Part model, mm, in its own coordinate system. Face numbers are marked on the shaded views. A direction names the side the tool comes from. Round coordinates to 2 decimals unless told otherwise and drop trailing zeros. Write each loop counter-clockwise with the first axis right and the second up, starting at its lowest first coordinate (ties: lowest second). Pieces come first, ordered by that corner, then holes. Notation, with made-up numbers: (-29, 78.5) -> (7, 78.5) arc R18 cw to (7, 104.5) -> close; hole circle Ø9 at (48, 11.25). An arc over 180 degrees is marked (long way). Return JSON: item names as keys, results as strings. Group by question number.
Autodesk Inventor part; units mm, degrees
ref_plane "YZ Plane" through (0, 0, 0) normal (1, 0, 0) x (0, 1, 0)
ref_plane "XZ Plane" through (0, 0, 0) normal (0, 1, 0) x (-1, 0, 0)
ref_plane "XY Plane" through (0, 0, 0) normal (0, 0, 1) x (1, 0, 0)
sketch "Эскиз1" plane through (0, 0, 0) normal (0, 1, 0) x (-1, 0, 0)
  line L0 (-40, 10) -> (40, 10)
  line L1 (40, 10) -> (40, -10)
  line L2 (40, -10) -> (-40, -10)
  line L3 (-40, -10) -> (-40, 10)
  line L4 (-40, 10) -> (40, -10) construction
  line L5 (40, 10) -> (-40, -10) construction
  point P0 (0, 0)
  dimension "d0" = 80
  dimension "d1" = 20
extrude "Выдавливание1" add sketch "Эскиз1" along normal blind 1.6
sketch "Эскиз2" plane through (0, 1.6, 0) normal (0, 1, 0) x (1, 0, 0)
  line L0 (-37.5, -7.5) -> (-37.5, 7.5)
  line L1 (37.5, 7.5) -> (37.5, -7.5)
  circle A0 centre (-37.5, -7.5) radius 1.5
  circle A1 centre (-37.5, 7.5) radius 1.5
  circle A2 centre (37.5, 7.5) radius 1.5
  circle A3 centre (37.5, -7.5) radius 1.5
  point P0 (0, 0)
  dimension "d4" = 75
  dimension "d5" = 15
  dimension "d6" = 3
  dimension "d7" = 3
  dimension "d8" = 3
  dimension "d9" = 3
extrude "Выдавливание2" cut sketch "Эскиз2" against normal blind 1.6
sketch "Эскиз3" plane through (0, 1.6, 0) normal (0, 1, 0) x (1, 0, 0)
  line L0 (15, -5) -> (-15, -5)
  line L1 (-15, -5) -> (-15, 5)
  line L2 (-15, 5) -> (15, 5)
  line L3 (15, 5) -> (15, -5)
  line L4 (15, -5) -> (-15, 5) construction
  line L5 (-15, -5) -> (15, 5) construction
  point P0 (0, 0)
  dimension "d12" = 30
  dimension "d13" = 10
extrude "Выдавливание3" add sketch "Эскиз3" along normal blind 8
properties part number "КВ33.044.1003 - Плата контроля сервомоторами" material "Серебро"
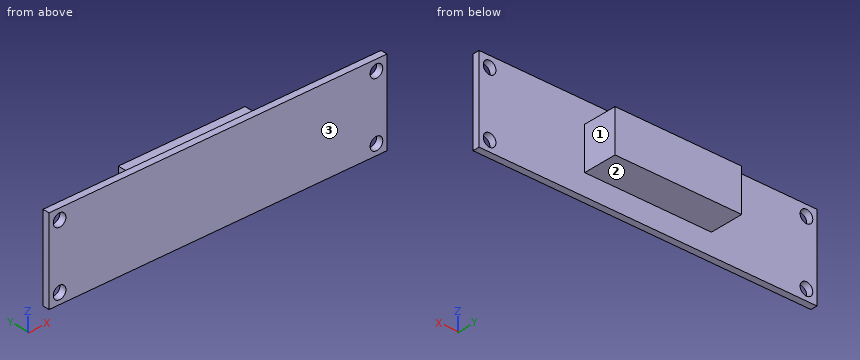
Item 1: Cut at B-B (x = 12.5). Write the cut outline in (y, z), then the cut area to 3 significant figures.
Item 2: Which spindle directions (+Z, -Z, +X, -X, +Y, -Y) get a long thin tool onto all of the face, cutting with end or side? Do the marked faces 1, 2 and 3. Say none if no direction does.
Item 3: Wall check: L1, parallel to Z at x = 37.5, y = 1.1; L2, parallel to X at y = 0.65, z = 7.5; L3, parallel to Y at x = -16, z = 9. Give the ranges that are in metal, low to high.
Item 4: Cut at A-A (z = -7.5). Write the cut outline in (x, y), then the cut area to 3 significant figures.
Item 5: Flat gauge pins, fed straight in: P1, Ø5, axis at x = -37.5, z = -7.5, coming from the +Y side; P2, Ø4, axis at x = 0.5, y = 7, coming from the -Z side; P3, Ø4, axis at x = -2, y = 5, coming from the +Z side. Where does each tip first touch, or does it go through?
Item 6: Cut at D-D (z = 2). Write the cut outline in (x, y).
Item 7: Cut at C-C (x = -37.5). Write the cut outline in (y, z).
Checks:
{
 "1": {"outline": "(0, -10) -> (1.6, -10) -> (1.6, -5) -> (9.6, -5) -> (9.6, 5) -> (1.6, 5) -> (1.6, 10) -> (0, 10) -> close", "area": "112 mm2"},
 "2": {"face 1": "+Z, -Z, +X, +Y", "face 2": "-Z, +X, -X, +Y", "face 3": "+Z, -Z, +X, -X, -Y"},
 "3": {"L1": "z = -10 to -9, -6 to 6, 9 to 10", "L2": "x = -40 to -39, -36 to 36, 39 to 40", "L3": "y = 0 to 1.6"},
 "4": {"outline": "(-40, 0) -> (-39, 0) -> (-39, 1.6) -> (-40, 1.6) -> close; (-36, 0) -> (36, 0) -> (36, 1.6) -> (-36, 1.6) -> close; (39, 0) -> (40, 0) -> (40, 1.6) -> (39, 1.6) -> close", "area": "118 mm2"},
 "5": {"P1": "stops at y = 1.6", "P2": "stops at z = -5", "P3": "stops at z = 5"},
 "6": {"outline": "(-40, 0) -> (40, 0) -> (40, 1.6) -> (15, 1.6) -> (15, 9.6) -> (-15, 9.6) -> (-15, 1.6) -> (-40, 1.6) -> close"},
 "7": {"outline": "(0, -10) -> (1.6, -10) -> (1.6, -9) -> (0, -9) -> close; (0, -6) -> (1.6, -6) -> (1.6, 6) -> (0, 6) -> close; (0, 9) -> (1.6, 9) -> (1.6, 10) -> (0, 10) -> close"}
}
